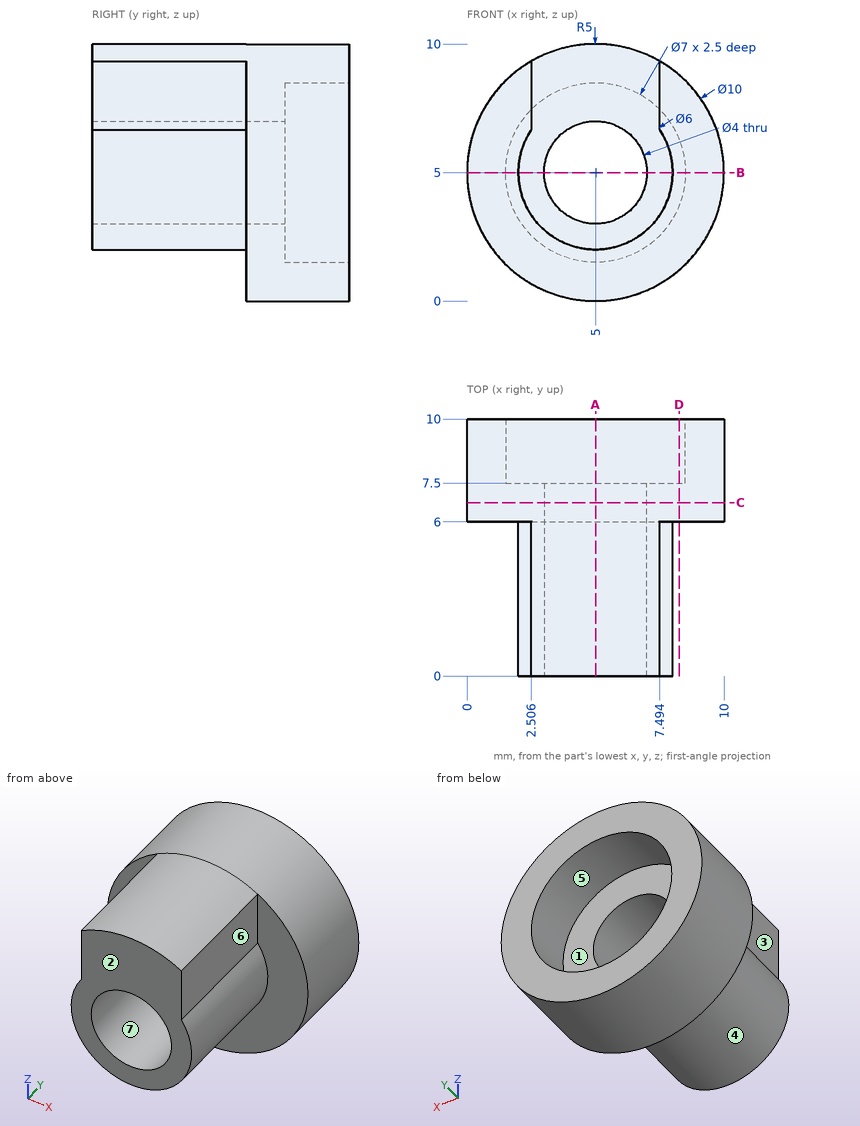
Check sheet for the drawn part. Datum: minimum x, y, z corner. Units: mm. A direction names the side the tool comes from. Give positions to 0.01 mm unless a question says otherwise; leave off trailing zeros. Write each loop counter-clockwise with the first axis right and the second up, starting at its lowest first coordinate (ties: lowest second). Pieces come first, ordered by that corner, then holes. Notation, with made-up numbers: M 80.25,-10.5 L 110.25,-10.5 A28 ccw 110.25,17.5 Z; hole C 23.25,60 d10. An arc over 180 degrees is marked long. One line per question, with ' | ' between items.
1. Gauge pin test, flat ends, axial feed: pin 1 (3.5 mm diameter, centred on x = 5, z = 5, fed in from +Y); pin 2 (1.3 mm diameter, centred on y = 2.5, z = 7.5, fed in from +X); pin 3 (1 mm diameter, centred on x = 8.5, z = 8.5, fed in from -Y); pin 4 (2 mm diameter, centred on x = 7, y = 8.5, fed in from +Z). Record the tip position at first contact, or that the pin passes through.
Ans:
pin 1: through | pin 2: x = 7.49 | pin 3: y = 6 | pin 4: z = 9.9
2. Scan lines: line 1 along Z through (x, y) = (5, 9.3); line 2 along Z through (x, y) = (5.25, 7) (1 decimal); line 3 along Y through (x, z) = (8, 8.5). Record each from-to range of solid material in increasing order. Write a range as from..to.
Ans:
line 1: 0..1.5, 8.5..10 | line 2: 0..3, 7..10 | line 3: 6..10
3. Mould release check, pull along Z, two halves, no side actions. Record for the marked faces 4, 5, 6 and 7: released by +Z, released by -Z, zero draft, split by the parting line, or undercut.
Ans:
face 4: split by the parting line | face 5: undercut | face 6: zero draft | face 7: undercut
4. Cross-section at B-B (z = 5). Enter the section's corners in (x, y).
Ans:
outline: M 0,6 L 2,6 L 2,0 L 3,0 L 3,7.5 L 1.5,7.5 L 1.5,10 L 0,10 Z; M 7,0 L 8,0 L 8,6 L 10,6 L 10,10 L 8.5,10 L 8.5,7.5 L 7,7.5 Z
5. Cross-section at D-D (x = 8.25). Enter the section's corners in (y, z), plus the area to 3 significant figures.
Ans:
outline: M 6,1.2 L 10,1.2 L 10,3.7 L 7.5,3.7 L 7.5,6.3 L 10,6.3 L 10,8.8 L 6,8.8 Z | area: 23.9 mm2
6. Set-up check for the marked faces 1, 2 and 3: record each of +Z, -Z, +X, -X, +Y, -Y from which the full face is reachable in a straight line by a thin tool's end or side.
Ans:
face 1: +Y | face 2: +Z, -Z, +X, -X, -Y | face 3: +Z, -X, -Y
7. Cross-section at A-A (x = 5). Enter the section's corners in (y, z), plus the area to 3 significant figures.
Ans:
outline: M 0,2 L 6,2 L 6,0 L 10,0 L 10,1.5 L 7.5,1.5 L 7.5,3 L 0,3 Z; M 0,7 L 7.5,7 L 7.5,8.5 L 10,8.5 L 10,10 L 0,10 Z | area: 40.5 mm2
8. Cross-section at C-C (y = 6.75). Enter the section's corners in (x, z).
Ans:
outline: C 5,5 d10; hole C 5,5 d4
